Read the model definition and answer for the solid it produces. Units are mm, in the model's axes. Give positions to 0.01 mm unless a question says otherwise; leave off trailing zeros. Write each loop counter-clockwise with the first axis right and the second up, starting at its lowest first coordinate (ties: lowest second). Pieces come first, ordered by that corner, then holes. Notation, with made-up numbers: (8, -14) -> (33, -14) arc R22 ccw to (33, 13) -> close; hole circle Ø1 at (20.5, 78). An arc over 180 degrees is marked (long way). Write item = value, one per line.
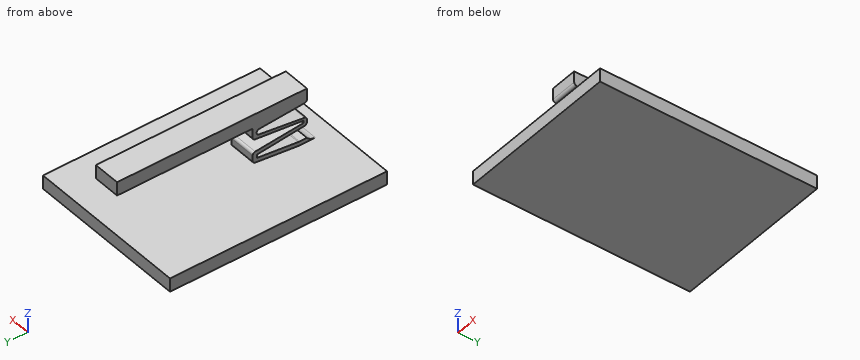
from build123d import *

# Parameters (mm, degrees)
F0_W        = 76.2
F0_H        = 101.6
F1_DEPTH    = 6.35
F2_W        = 12.7
F2_H        = 25.4
F3_DEPTH    = 25.4
F4_W        = 63.5
F4_H        = 6.35
F5_DEPTH    = 12.7
F7_DEPTH    = 12.7
F8_T1_DEPTH = 12.7
F9_R        = 1.27


# Not quite as in the source:
# - a fillet or chamfer that OpenCascade refuses, or shapes differently, is made with other operations: its cross-section is extruded or revolved along the edge and cut away or added


with BuildPart() as f1:
    # F0 (on Top) → F1 (new body)
    with BuildSketch(Plane.XY):
        Rectangle(F0_W, F0_H)
    extrude(amount=-F1_DEPTH)

    # F2 (on face) → F3 (join)
    with BuildSketch(Plane.XY):
        with Locations((0, -25.4)):
            Rectangle(F2_W, F2_H)
    extrude(amount=F3_DEPTH)

    # F4 (on face) → F5 (join, through all)
    with BuildSketch(Plane.YZ.offset(6.35)):
        with Locations((19.05, 22.225)):
            Rectangle(F4_W, F4_H)
    extrude(amount=-F5_DEPTH)

    # F6 (on face) → F7 (cut, through all)
    with BuildSketch(Plane.YZ.offset(6.35)):
        Polygon((-12.7, 2.3706669454), (-33.9936651289, 0), (-12.7, 0), align=None)
        Polygon((-38.1, 1.8626668025), (-34.33233127, 1.8626668025), (-14.6236953676, 4.0568692279), (-14.6236953676, 5.64925652), (-38.1, 8.2224374637), align=None)
        Polygon((-36.4234596491, 9.7253257409), (-12.7, 7.3805158027), (-12.7, 13.4764490649), (-36.4234596491, 10.8793787658), align=None)
        Polygon((-38.1, 19.05), (-38.1, 11.84564922), (-14.5409666002, 14.9470388849), (-14.5409666002, 17.2827038914), align=None)
    extrude(amount=-F7_DEPTH, mode=Mode.SUBTRACT)

    # F8: fillet of radius 5.08 on 2 edges, made by hand

    # F8_s2 → F8_t1 (join)
    with BuildSketch(Plane.YZ.offset(-6.35)):
        with BuildLine():
            ThreePointArc((-42.0313060293, 0), (-39.8561799, 0.4892237779), (-38.1, 1.8626668025))
            Line((-38.1, 1.8626668025), (-38.1, 0))
            Line((-38.1, 0), (-42.0313060293, 0))
        make_face()
        with BuildLine():
            ThreePointArc((-34.6142437504, 1.8626668025), (-34.3327643656, 1.870471089), (-34.0521498413, 1.8938599694))
            Line((-34.0521498413, 1.8938599694), (-34.33233127, 1.8626668025))
            Line((-34.33233127, 1.8626668025), (-34.6142437504, 1.8626668025))
        make_face()
    extrude(amount=F8_T1_DEPTH)

    # F9
    f9_edges = [f1.edges().sort_by_distance(p)[0] for p in [
        (0, -12.7, 7.380516),
        (0, -12.7, 2.370667),
        (0, -38.1, 11.845649),
        (0, -38.1, 8.222437),
        (0, -12.7, 13.476449),
        (0, -38.1, 19.05),
        (0, -14.540967, 17.282704),
        (0, -14.540967, 14.947039),
    ]]
    fillet(f9_edges, radius=F9_R)


solid = f1.part
(1) Given P1, Ø1, axis at x = -25.5, y = 36, coming from the +Z side; P2, Ø7.5, axis at y = -10.5, z = 7, coming from the +X side; P3, Ø0.6, axis at x = -2.5, z = 10.5, coming from the +Y side, each flat-ended and moving along its own axis, determine where each tip first touches the part or whether it passes through.
Checks:
P1 = 0
P2 = 6.35
P3 = -36.42
(2) The part is cut by section D-D on x = -25.5. Determine the outline of the cut face in (y, z).
Checks:
outline = (-50.8, -6.35) -> (50.8, -6.35) -> (50.8, 0) -> (-50.8, 0) -> close
(3) The part is cut by section B-B on y = 44. Determine the outline of the cut face in (x, z).
Checks:
outline = (-38.1, -6.35) -> (38.1, -6.35) -> (38.1, 0) -> (-38.1, 0) -> close; (-6.35, 19.05) -> (6.35, 19.05) -> (6.35, 25.4) -> (-6.35, 25.4) -> close
(4) Consider L1, parallel to Z at x = 1, y = 10; L2, parallel to Z at x = -4, y = -20; L3, parallel to Z at x = -24, y = -39.5. Determine where each line is inside the solid, lowest interval first.
Checks:
L1 = -6.35 to 0, 19.05 to 25.4
L2 = -6.35 to 0, 1.56 to 3.46, 6.24 to 8.1, 12.68 to 14.23, 17.69 to 25.4
L3 = -6.35 to 0
(5) The part is cut by section C-C on y = -32. Determine the outline of the cut face in (x, z), plus the area to 3 significant figures.
Checks:
outline = (-38.1, -6.35) -> (38.1, -6.35) -> (38.1, 0) -> (-38.1, 0) -> close; (-6.35, 0.22) -> (6.35, 0.22) -> (6.35, 2.12) -> (-6.35, 2.12) -> close; (-6.35, 7.55) -> (6.35, 7.55) -> (6.35, 9.29) -> (-6.35, 9.29) -> close; (-6.35, 11.36) -> (6.35, 11.36) -> (6.35, 12.65) -> (-6.35, 12.65) -> close; (-6.35, 18.59) -> (6.35, 18.59) -> (6.35, 25.4) -> (-6.35, 25.4) -> close
area = 633 mm²
